For this review, take the finished solid that the model builds, in its own axes (mm). A direction names the side the tool comes from. Coordinates: 2 decimals unless noted, no trailing zeros. Loops run counter-clockwise (first coordinate to the right, second up) from the corner with the lowest first, then second, coordinate; pieces in that order, holes last. Notation, with made-up numbers: (33, -0.75) - (52, -0.75) arc R15 cw to (52, 5.25) - close; hole circle Ø2 at (-35.5, 21). An arc over 180 degrees is marked (long way). Answer as a JSON object with one key per item and string values. Group by question number.
Item 1: Tool access review of faces 1 (the flat face through (7, 9, 2)), 2 (the cylindrical face through (0.86, 0.9, 0.76)): name each direction out of +Z, -Z, +X, -X, +Y, -Y from which nothing blocks a thin tool from reaching the whole face with its end or side.
Item 2: We need section D-D (x = 17.25). Give the boundary of the cut face in (y, z).
Item 3: To check wall thickness, follow line 1 (Y direction, x = 8.75, z = 2) (3 decimals); line 2 (Z direction, x = 17.25, y = 11.25); line 3 (X direction, y = 10, z = 2.15). State the ranges of each line that lie inside material, in increasing order.
Item 4: We need section B-B (y = 17.95). Give the boundary of the cut face in (x, z).
Item 5: We need section C-C (z = 0.95). Give the boundary of the cut face in (x, y), then the cut area to 3 significant figures.
Item 6: Clearance check with flat-ended pins moving along their axes: pin 1 (5 mm diameter, centred on x = 14.5, y = 11, fed in from +Z); pin 2 (1.2 mm diameter, centred on x = 7.5, z = 2.5, fed in from +Y); pin 3 (4 mm diameter, centred on x = 17.76, y = 17.95, fed in from +Z); pin 4 (2 mm diameter, centred on x = 2.74, y = 17.95, fed in from +Z). State where each tip first meets the part, or that it passes through.
Item 7: Mouldability with a two-part tool opening along X and no side actions: class faces 3 (the flat face through (7, 7, 2.5)), 4 (the cylindrical face through (5.933, 8.215, 1.993)), 5 (the cylindrical face through (19.64, 19.6, 0.76)) as released by +X, released by -X, zero draft, split by the parting line, or undercut.
Item 8: We need section A-A (z = 2.05). Give the boundary of the cut face in (x, y) (3 decimals).
from build123d import *

# Parameters (mm, degrees)
SKETCH1_W           = 20.5
SKETCH1_H           = 20.5
BOSS_EXTRUDE1_DEPTH = 1.5
FILLET1_R           = 3
SKETCH9_R           = 1.25
CUT_EXTRUDE1_DEPTH  = 4.5
SKETCH10_W          = 2.5
SKETCH10_H          = 2.5
BOSS_EXTRUDE2_DEPTH = 0.8
SKETCH11_W          = 2
SKETCH11_H          = 2.75
BOSS_EXTRUDE3_DEPTH = 1.5
SKETCH12_R          = 4
SKETCH12_R_2        = 3.55
BOSS_EXTRUDE4_DEPTH = 1


with BuildPart() as part:
    # Sketch1 → Boss-Extrude1 (new body)
    with BuildSketch(Plane.XY):
        with Locations((10.25, 10.25)):
            Rectangle(SKETCH1_W, SKETCH1_H)
    extrude(amount=BOSS_EXTRUDE1_DEPTH)

    # Fillet1
    fillet1_edges = [part.edges().sort_by_distance(p)[0] for p in [
        (0, 20.5, 0.75),
        (20.5, 20.5, 0.75),
        (20.5, 0, 0.75),
        (0, 0, 0.75),
    ]]
    fillet(fillet1_edges, radius=FILLET1_R)

    # Sketch9 → Cut-Extrude1 (cut)
    with BuildSketch(Plane.XY.offset(1.5)):
        with Locations((17.762103221, 17.95)):
            Circle(SKETCH9_R)
        with Locations((2.737896779, 17.95)):
            Circle(SKETCH9_R)
    extrude(amount=-CUT_EXTRUDE1_DEPTH, mode=Mode.SUBTRACT)

    # Sketch10 → Boss-Extrude2 (add)
    with BuildSketch(Plane.XY.offset(1.5)):
        with Locations((10.25, 10.25)):
            Rectangle(SKETCH10_W, SKETCH10_H)
    extrude(amount=BOSS_EXTRUDE2_DEPTH)

    # Sketch11 → Boss-Extrude3 (add)
    with BuildSketch(Plane.XY.offset(1.5)):
        with Locations((7, 10.375)):
            Rectangle(SKETCH11_W, SKETCH11_H)
    extrude(amount=BOSS_EXTRUDE3_DEPTH)

    # Sketch12 → Boss-Extrude4 (add)
    with BuildSketch(Plane.XY.offset(1.5)):
        with Locations((8.75, 10.375)):
            Circle(SKETCH12_R)
        with Locations((8.75, 10.375)):
            Circle(SKETCH12_R_2, mode=Mode.SUBTRACT)
    extrude(amount=BOSS_EXTRUDE4_DEPTH)


solid = part.part
Check sheet entries:
{
 "1": {"face 1": "+Z", "face 2": "+Z, -Z, -X, -Y"},
 "2": {"outline": "(0, 0) - (16.81, 0) - (16.81, 1.5) - (0, 1.5) - close; (19.09, 0) - (20.5, 0) - (20.5, 1.5) - (19.09, 1.5) - close"},
 "3": {"line 1": "y = 6.375 to 6.825, 13.925 to 14.375", "line 2": "z = 0 to 1.5", "line 3": "x = 4.77 to 5.22, 6 to 8, 9 to 11.5, 12.28 to 12.73"},
 "4": {"outline": "(0.03, 0) - (1.49, 0) - (1.49, 1.5) - (0.03, 1.5) - close; (3.99, 0) - (16.51, 0) - (16.51, 1.5) - (3.99, 1.5) - close; (19.01, 0) - (20.47, 0) - (20.47, 1.5) - (19.01, 1.5) - close"},
 "5": {"outline": "(0, 3) arc R3 ccw to (3, 0) - (17.5, 0) arc R3 ccw to (20.5, 3) - (20.5, 17.5) arc R3 ccw to (17.5, 20.5) - (3, 20.5) arc R3 ccw to (0, 17.5) - close; hole circle Ø2.5 at (2.74, 17.95); hole circle Ø2.5 at (17.76, 17.95)", "area": "403 mm2"},
 "6": {"pin 1": "stops at z = 2.5", "pin 2": "stops at y = 14.32", "pin 3": "stops at z = 1.5", "pin 4": "passes through"},
 "7": {"face 3": "zero draft", "face 4": "undercut", "face 5": "released by +X"},
 "8": {"outline": "circle Ø8 at (8.75, 10.375); (6, 9) - (8, 9) - (8, 11.75) - (6, 11.75) - close; (9, 9) - (11.5, 9) - (11.5, 11.5) - (9, 11.5) - close; hole circle Ø7.1 at (8.75, 10.375)"}
}
